Check sheet for the modelled part. Datum: model origin and axes. Units: mm. Round coordinates to 2 decimals unless told otherwise and drop trailing zeros. Write each loop counter-clockwise with the first axis right and the second up, starting at its lowest first coordinate (ties: lowest second). Pieces come first, ordered by that corner, then holes.
Item 1: Section check B-B, the plane z = -10.16. Record the cut outline in (x, y), plus the area to 3 significant figures.
Item 2: Release check for a two-part mould opening along X. For faces 1 (the flat face through (-12.7, 0.5, 0.2)), 2 (the flat face through (12.7, 0.5, -0.2)), 3 (the cylindrical face through (-10.03, 0.49, 9.17)) record: pulls with the +X half, pulls with the -X half, needs draft (parallel to the pull), parting line crosses it, or undercut.
Item 3: Section check A-A, the plane y = 0.7. Record the cut outline in (x, z).
Item 4: Section check C-C, the plane x = 10.16. Record the cut outline in (y, z).
Item 5: Depth check by flat-ended pin: pin 1 (1.8 mm diameter, centred on x = -10.16, z = 10.16, fed in from -Y). Enter the tip coordinate at first touch or a pass-through.
Item 6: Material ranges on line 1 along Z through (x, y) = (-10.16, 0.3); line 2 along X through (y, z) = (0.5, 10.5); line 3 along X through (y, z) = (0.9, -9.5), recorded low to high.
Autodesk Inventor part; units mm, degrees
ref_plane "YZ Plane" through (0, 0, 0) normal (1, 0, 0) x (0, 1, 0)
ref_plane "XZ Plane" through (0, 0, 0) normal (0, 1, 0) x (-1, 0, 0)
ref_plane "XY Plane" through (0, 0, 0) normal (0, 0, 1) x (1, 0, 0)
sketch "Sketch1" plane through (0, 0, 0) normal (0, 1, 0) x (-1, 0, 0)
  line L0 (-12.7, 12.7) -> (12.7, 12.7)
  line L1 (12.7, 12.7) -> (12.7, -12.7)
  line L2 (12.7, -12.7) -> (-12.7, -12.7)
  line L3 (-12.7, -12.7) -> (-12.7, 12.7)
  line L4 (-12.7, 12.7) -> (12.7, -12.7) construction
  line L5 (12.7, 12.7) -> (-12.7, -12.7) construction
  circle A0 centre (10.16, 10.16) radius 1
  line L6 (0, 15.3102) -> (0, -24.4188) construction
  line L7 (16, 0) -> (-15.6009, 0) construction
  circle A1 centre (10.16, -10.16) radius 1
  circle A2 centre (-10.16, 10.16) radius 1
  circle A3 centre (-10.16, -10.16) radius 1
  point P0 (0, 0)
  dimension "d0" = 25.4
  dimension "d1" = 25.4
  dimension "d2" = 2.54
  dimension "d3" = 2.54
extrude "Extrusion1" add sketch "Sketch1" along normal blind 1
properties part number "step_down_Suba"
Values found:
1. outline: (-12.7, 0) - (-11.16, 0) - (-11.16, 1) - (-12.7, 1) - close; (-9.16, 0) - (9.16, 0) - (9.16, 1) - (-9.16, 1) - close; (11.16, 0) - (12.7, 0) - (12.7, 1) - (11.16, 1) - close
1. area: 21.4 mm2
2. face 1: pulls with the -X half
2. face 2: pulls with the +X half
2. face 3: undercut
3. outline: (-12.7, -12.7) - (12.7, -12.7) - (12.7, 12.7) - (-12.7, 12.7) - close; hole circle Ø2 at (-10.16, -10.16); hole circle Ø2 at (-10.16, 10.16); hole circle Ø2 at (10.16, -10.16); hole circle Ø2 at (10.16, 10.16)
4. outline: (0, -12.7) - (1, -12.7) - (1, -11.16) - (0, -11.16) - close; (0, -9.16) - (1, -9.16) - (1, 9.16) - (0, 9.16) - close; (0, 11.16) - (1, 11.16) - (1, 12.7) - (0, 12.7) - close
5. pin 1: passes through
6. line 1: z = -12.7 to -11.16, -9.16 to 9.16, 11.16 to 12.7
6. line 2: x = -12.7 to -11.1, -9.22 to 9.22, 11.1 to 12.7
6. line 3: x = -12.7 to -10.91, -9.41 to 9.41, 10.91 to 12.7
